Geometry: final body of the model. Coordinates: model frame, mm. Face numbers are marked on the shaded views. A direction names the side the tool comes from. Give positions to 0.01 mm unless a question says otherwise; leave off trailing zeros. Loops run counter-clockwise (first coordinate to the right, second up) from the corner with the lowest first, then second, coordinate; pieces in that order, holes last.
from build123d import *

# Parameters (mm, degrees)
PAD_DEPTH    = 28
SKETCH002_W  = 2.838082
SKETCH002_H  = 27.969857
PAD001_DEPTH = 2
FILLET_R     = 1
SKETCH003_W  = 2.802156
SKETCH003_H  = 27.921276
PAD002_DEPTH = 2
FILLET001_R  = 1
FILLET002_R  = 1
FILLET003_R  = 1
FILLET004_R  = 1


with BuildPart() as part:
    # Sketch001 → Pad (new body)
    with BuildSketch(Plane.XY):
        Polygon((7.12948, 20.78117), (7.445243, 21.187149), (7.854891, 21.607611), (8.508251, 22.283501), (9.696487, 23.44212), (10.384461, 23.44212), (12.655314, 21.14204), (12.798072, 20.62591), (12.798072, 19.983595), (12.798072, 19.585785), (10.85096, 19.585785), (10.85096, 17.475296), (10.85096, 14.854997), (10.85096, -19.505323), (12.701512, -19.51746), (12.724067, -20.600073), (12.521076, -21.321814), (10.456077, -23.362608), (10.24308, -23.464483), (9.610203, -23.458431), (7.33356, -21.163933), (7.172753, -20.632019), (7.013088, -20.473427), (6.702209, -20.340731), (3.07281, -20.340731), (3.07281, -27.006718), (14.752544, -27.006718), (14.752544, 25.795757), (3.011012, 25.795757), (3.011012, 20.555626), (7.106926, 20.555626), align=None)
    extrude(amount=PAD_DEPTH)

    # Sketch002 → Pad001 (new body)
    with BuildSketch(Plane.YZ.offset(14.752544)):
        with Locations((-19.919058, 13.984928)):
            Rectangle(SKETCH002_W, SKETCH002_H)
    extrude(amount=PAD001_DEPTH)

    # Fillet
    fillet_edges = [part.edges().sort_by_distance(p)[0] for p in [
        (16.752544, -19.919058, 27.969857),
        (16.752544, -18.500017, 13.984929),
        (16.752544, -19.919058, 0),
        (16.752544, -21.338099, 13.984929),
    ]]
    fillet(fillet_edges, radius=FILLET_R)

    # Sketch003 → Pad002 (new body)
    with BuildSketch(Plane.YZ.offset(14.752544)):
        with Locations((20.083518, 13.960638)):
            Rectangle(SKETCH003_W, SKETCH003_H)
    extrude(amount=PAD002_DEPTH)

    # Fillet001
    fillet001_edges = [part.edges().sort_by_distance(p)[0] for p in [
        (16.752544, 20.083518, 27.921276),
        (16.752544, 21.484596, 13.960638),
        (16.752544, 20.083518, 0),
        (16.752544, 18.68244, 13.960638),
    ]]
    fillet(fillet001_edges, radius=FILLET001_R)

    # Fillet002
    fillet002_edges = [part.edges().sort_by_distance(p)[0] for p in [
        (3.07281, -27.006718, 14),
        (14.752544, -27.006718, 14),
        (8.912677, -27.006718, 0),
        (8.912677, -27.006718, 28),
    ]]
    fillet(fillet002_edges, radius=FILLET002_R)

    # Fillet003
    fillet003_edges = [part.edges().sort_by_distance(p)[0] for p in [
        (14.752544, 25.795757, 14),
        (3.011012, 25.795757, 14),
        (8.881778, 25.795757, 0),
        (8.881778, 25.795757, 28),
    ]]
    fillet(fillet003_edges, radius=FILLET003_R)

    # Fillet004
    fillet004_edges = [part.edges().sort_by_distance(p)[0] for p in [
        (10.85096, 19.585785, 14),
        (10.85096, 0.040231, 0),
        (10.85096, -19.505323, 14),
        (10.85096, 0.040231, 28),
    ]]
    fillet(fillet004_edges, radius=FILLET004_R)


solid = part.part
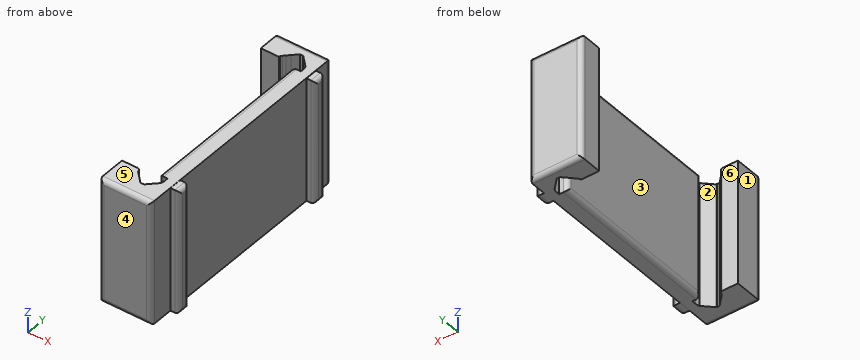
Item 1: Pin query (flat end, axial travel): pin 1 (1.1 mm diameter, centred on x = 15, z = 11, fed in from +Y); pin 2 (13 mm diameter, centred on y = 6.5, z = 8.5, fed in from -X); pin 3 (1.1 mm diameter, centred on x = 15.5, y = 20.5, fed in from +Z); pin 4 (5 mm diameter, centred on x = 5.5, y = 16, fed in from -Z). Return the tip coordinate at first contact, or that it passes through.
Values follow:
pin 1: stops at y = 25.51
pin 2: stops at x = 10.85
pin 3: stops at z = 27.92
pin 4: passes through
Item 2: Section query A-A on x = 6. Return loops of the section in (y, z).
Values follow:
outline: (-27.01, 1) arc R1 ccw to (-26.01, 0) - (-20.34, 0) - (-20.34, 28) - (-26.01, 28) arc R1 ccw to (-27.01, 27) - close; (20.56, 0) - (24.8, 0) arc R1 ccw to (25.8, 1) - (25.8, 27) arc R1 ccw to (24.8, 28) - (20.56, 28) - close
Item 3: Draft query along Y for the marked faces 4, 5 and 6. Return one class per face: +Y half, -Y half, draft (parallel to the pull), parting line (faces both ways), or undercut.
Values follow:
face 4: -Y half
face 5: draft
face 6: undercut
Item 4: Ray query, probe 1 along Y at (x, z) = (6, 5); probe 2 along Y at (x, z) = (15.75, 9.5); probe 3 along Y at (x, z) = (12.25, 3.5). Return the intervals inside material, ascending.
Values follow:
probe 1: y = -27.01 to -20.34, 20.56 to 25.8
probe 2: y = -21.34 to -18.5, 18.68 to 21.48
probe 3: y = -27.01 to -21.59, -19.51 to 19.59, 21.55 to 25.8
Item 5: Set-up query: the marked faces 1, 2 and 3. Return all of +Z, -Z, +X, -X, +Y, -Y with unobstructed straight access to the full face (end or side cutting, diameter ignored); none if empty.
Values follow:
face 1: +Z, -Z, -X, -Y
face 2: +Z, -Z
face 3: +Z, -Z, -X
Item 6: Section query B-B on y = -18. Return loops of the section in (x, z), plus the area to 3 significant figures.
Values follow:
outline: (10.85, 1) arc R1 ccw to (11.85, 0) - (14.75, 0) - (14.75, 28) - (11.85, 28) arc R1 ccw to (10.85, 27) - close
area: 109 mm2
